Read the model definition and answer for the solid it produces. Units are mm, in the model's axes. Face numbers are marked on the shaded views. A direction names the side the tool comes from. Coordinates: 2 decimals unless noted, no trailing zeros. Write each loop counter-clockwise with the first axis right and the second up, starting at its lowest first coordinate (ties: lowest second). Pieces come first, ordered by that corner, then holes.
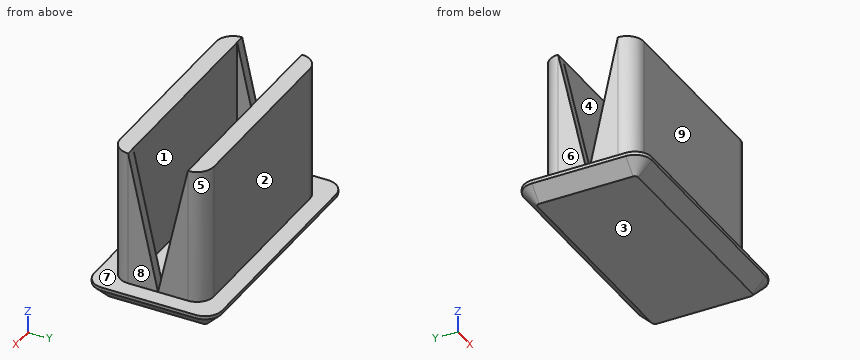
from build123d import *

# Parameters (mm, degrees)
F0_W     = 12.5
F0_H     = 5.5
F0_W_2   = 11.4
F0_H_2   = 3.5
F1_DEPTH = 8
F0_W_3   = 14.5
F0_H_3   = 7.5
F2_DEPTH = 1
F3_R     = 1
F5_DEPTH = 25
F6_SIZE  = 0.8


with BuildPart() as f1:
    # F0 (on Top) → F1 (new body)
    with BuildSketch(Plane.XY):
        with Locations((-11.856854585, 4.7651143782)):
            Rectangle(F0_W, F0_H)
        with Locations((-11.856854585, 4.7651143782)):
            Rectangle(F0_W_2, F0_H_2, mode=Mode.SUBTRACT)
    extrude(amount=F1_DEPTH)

    # F0 (on Top) → F2 (join)
    with BuildSketch(Plane.XY):
        with Locations((-11.856854585, 4.7651143782)):
            Rectangle(F0_W_3, F0_H_3)
        with Locations((-11.856854585, 4.7651143782)):
            Rectangle(F0_W, F0_H, mode=Mode.SUBTRACT)
        with Locations((-11.856854585, 4.7651143782)):
            Rectangle(F0_W, F0_H)
        with Locations((-11.856854585, 4.7651143782)):
            Rectangle(F0_W_2, F0_H_2, mode=Mode.SUBTRACT)
        with Locations((-11.856854585, 4.7651143782)):
            Rectangle(F0_W_2, F0_H_2)
    extrude(amount=-F2_DEPTH)

    # F3
    f3_edges = [f1.edges().sort_by_distance(p)[0] for p in [
        (-18.106855, 2.015114, 4),
        (-5.606855, 2.015114, 4),
        (-18.106855, 7.515114, 4),
        (-5.606855, 7.515114, 4),
        (-19.106855, 1.015114, -0.5),
        (-4.606855, 1.015114, -0.5),
        (-19.106855, 8.515114, -0.5),
        (-4.606855, 8.515114, -0.5),
    ]]
    fillet(f3_edges, radius=F3_R)

    # F4 (on face) → F5 (cut)
    with BuildSketch(Plane.YZ.offset(-5.606854585)):
        Polygon((6.5151143782, 8), (3.0151143782, 8), (4.7651143782, 0), align=None)
    extrude(amount=-F5_DEPTH, mode=Mode.SUBTRACT)

    # F6
    f6_edges = [f1.edges().sort_by_distance(p)[0] for p in [
        (-11.856855, 1.015114, -1),
        (-18.813961, 1.308008, -1),
        (-4.899748, 1.308008, -1),
        (-4.606855, 4.765114, -1),
        (-4.899748, 8.222221, -1),
        (-11.856855, 8.515114, -1),
        (-19.106855, 4.765114, -1),
        (-18.813961, 8.222221, -1),
    ]]
    chamfer(f6_edges, length=F6_SIZE)


solid = f1.part
Item 1: For the marked faces 5, 6, 7, 8 and 9, determine the directions among +Z, -Z, +X, -X, +Y, -Y from which every point of the face is accessible in a straight line to the end or side of a thin tool.
Item 2: Find the intervals of material crossed by probe 1 along Y at (x, z) = (-13.75, 0.25); probe 2 along X at (y, z) = (5.5, 1.25); probe 3 along Z at (x, y) = (-14.5, 5.5), in increasing order.
Item 3: The part is cut by section C-C (y = 2.25). Give the vertices of the cut face in (x, z).
Item 4: The part is cut by section D-D (z = 6.75). Give the vertices of the cut face in (x, y), and give its area (3 significant figures).
Item 5: Given pin 1 (1.4 mm diameter, centred on y = 4.5, z = 4, fed in from +X); pin 2 (2 mm diameter, centred on x = -10, z = 5, fed in from -Y); pin 3 (1.4 mm diameter, centred on y = 4, z = 3.5, fed in from -X), each flat-ended and moving along its own axis, determine where each tip first touches the part or whether it passes through.
Item 6: The part is cut by section A-A (x = -9.5). Give the vertices of the cut face in (y, z).
Item 7: Determine the mould class of the marked faces 1, 2, 3 and 4 for opening direction Y: +Y half, -Y half, draft (parallel to the pull), parting line (faces both ways), or undercut.
Item 8: The part is cut by section B-B (z = 2.25). Give the vertices of the cut face in (x, y), and give its area (3 significant figures).
Answer:
1. face 5: +Z, +X, +Y
1. face 6: +Z, -X, +Y, -Y
1. face 7: +Z
1. face 8: +Z, +X, +Y, -Y
1. face 9: +Z, +X, -X, -Y
2. probe 1: y = 2.02 to 3.02, 6.52 to 7.52
2. probe 2: x = -18.11 to -17.56, -6.16 to -5.61
2. probe 3: z = -1 to 0
3. outline: (-19.11, -0.2) - (-18.31, -1) - (-5.41, -1) - (-4.61, -0.2) - (-4.61, 0) - (-5.96, 0) - (-5.96, 8) - (-17.75, 8) - (-17.75, 0) - (-19.11, 0) - close
4. outline: (-18.11, 3.02) arc R1 ccw to (-17.11, 2.02) - (-6.61, 2.02) arc R1 ccw to (-5.61, 3.02) - (-5.61, 3.29) - (-6.16, 3.29) - (-6.16, 3.02) - (-17.56, 3.02) - (-17.56, 3.29) - (-18.11, 3.29) - close; (-18.11, 6.24) - (-17.56, 6.24) - (-17.56, 6.52) - (-6.16, 6.52) - (-6.16, 6.24) - (-5.61, 6.24) - (-5.61, 6.52) arc R1 ccw to (-6.61, 7.52) - (-17.11, 7.52) arc R1 ccw to (-18.11, 6.52) - close
4. area: 24.7 mm2
5. pin 1: stops at x = -5.61
5. pin 2: stops at y = 2.02
5. pin 3: stops at x = -18.11
6. outline: (1.02, -0.2) - (1.82, -1) - (7.72, -1) - (8.52, -0.2) - (8.52, 0) - (7.52, 0) - (7.52, 8) - (6.52, 8) - (6.52, 0) - (3.02, 0) - (3.02, 8) - (2.02, 8) - (2.02, 0) - (1.02, 0) - close
7. face 1: undercut
7. face 2: +Y half
7. face 3: draft
7. face 4: undercut
8. outline: (-18.11, 3.02) arc R1 ccw to (-17.11, 2.02) - (-6.61, 2.02) arc R1 ccw to (-5.61, 3.02) - (-5.61, 4.27) - (-6.16, 4.27) - (-6.16, 3.02) - (-17.56, 3.02) - (-17.56, 4.27) - (-18.11, 4.27) - close; (-18.11, 5.26) - (-17.56, 5.26) - (-17.56, 6.52) - (-6.16, 6.52) - (-6.16, 5.26) - (-5.61, 5.26) - (-5.61, 6.52) arc R1 ccw to (-6.61, 7.52) - (-17.11, 7.52) arc R1 ccw to (-18.11, 6.52) - close
8. area: 26.9 mm2
